CAD build for the part. Positions are in the model's coordinates, mm. Face numbers are marked on the shaded views. A direction names the side the tool comes from. Coordinates: 2 decimals unless noted, no trailing zeros. Order: outer loops, then holes, each group sorted by start corner. A loop starts at its lowest first (then second) coordinate and runs counter-clockwise, first axis right, second up. Notation, with made-up numbers: (-24, 86.5) - (30, 86.5) arc R17 ccw to (30, 108.5) - close; hole circle Ø1 at (-3.5, 30). An arc over 180 degrees is marked (long way). Write each question's results on one line, items separated by ' | '. Start each with the question number.
Q1. Which spindle directions (+Z, -Z, +X, -X, +Y, -Y) get a long thin tool onto all of the face, cutting with end or side? Do the marked faces 4, 5, 6, 7 and 8. Say none if no direction does.
Q2. Wall check: probe 1 along Y at (x, z) = (-32, 22.5); probe 2 along Z at (x, y) = (47, -12.5); probe 3 along X at (y, z) = (9, 4). Give the ranges that are in metal, low to high.
Q3. Pin check, flat tips, straight feed: P1, Ø20.5, axis at x = 36.5, y = -8.5, coming from the +Z side; P2, Ø5.5, axis at x = 15, z = 40, coming from the -Y side; P3, Ø5, axis at x = 22.5, z = 38, coming from the +Y side. Stop position of each tip, or through.
Q4. Band-saw the part on B-B, the plane y = -38. Write the cut outline in (x, z), then the cut area to 3 significant figures.
Q5. Band-saw the part on C-C, the plane z = 7. Count the separate pieces of the cut face and the enclosed holes in it, then the cut area to 3 significant figures.
Q6. Band-saw the part on A-A, the plane x = 12. Write the cut outline in (y, z) (3 decimals), then the cut area to 3 significant figures.
Q7. Pull direction X, two halves, no side cores. Call the marked faces 1, 2 and 3: released by +X, released by -X, zero draft, split by the parting line, or undercut.
Q8. Band-saw the part on D-D, the plane z = 82. Write the cut outline in (x, y).
```python
from build123d import *

# Parameters (mm, degrees)
F0_W         = 101.6
F0_H         = 76.2
F1_DEPTH     = 25.4
F2_R         = 15.875
F3_R         = 15.875
F4_R         = 15.875
F5_R         = 15.875
F7_D         = 15.875
F8_SIZE      = 6.35
F9_W         = 19.05
F9_H         = 63.5
F10_DEPTH    = 69.85
F12_DEPTH    = 25.4
F13_T1_DEPTH = 156.5315328508
F14_T1_DEPTH = 156.5315328508


# Not quite as in the source:
# - a fillet or chamfer that OpenCascade refuses, or shapes differently, is made with other operations: its cross-section is extruded or revolved along the edge and cut away or added


with BuildPart() as f1:
    # F0 (on Top) → F1 (new body)
    with BuildSketch(Plane.XY):
        with Locations((6.2353381336, -17.6054243982)):
            Rectangle(F0_W, F0_H)
    extrude(amount=F1_DEPTH)

    # F2
    f2_edges = [f1.edges().sort_by_distance(p)[0] for p in [
        (57.035338, -55.705424, 12.7),
    ]]
    fillet(f2_edges, radius=F2_R)

    # F3
    f3_edges = [f1.edges().sort_by_distance(p)[0] for p in [
        (-44.564662, -55.705424, 12.7),
    ]]
    fillet(f3_edges, radius=F3_R)

    # F4
    f4_edges = [f1.edges().sort_by_distance(p)[0] for p in [
        (-44.564662, 20.494576, 12.7),
    ]]
    fillet(f4_edges, radius=F4_R)

    # F5
    f5_edges = [f1.edges().sort_by_distance(p)[0] for p in [
        (57.035338, 20.494576, 12.7),
    ]]
    fillet(f5_edges, radius=F5_R)

    # F7 (through all)
    with Locations(Plane(origin=(0, 0, 0), x_dir=(1, 0, 0), z_dir=(0, 0, -1))):
        with Locations((-28.6896618664, 39.8304243982), (41.1603381336, 39.8304243982), (41.1603381336, -4.6195756018), (-28.6896618664, -4.6195756018)):
            Hole(F7_D / 2)

    # F8
    f8_edges = [f1.edges().sort_by_distance(p)[0] for p in [
        (6.235338, -55.705424, 25.4),
        (6.235338, 20.494576, 25.4),
        (52.385658, 15.844896, 25.4),
        (-39.914982, 15.844896, 25.4),
        (57.035338, -17.605424, 25.4),
        (-44.564662, -17.605424, 25.4),
        (52.385658, -51.055745, 25.4),
        (-39.914982, -51.055745, 25.4),
    ]]
    chamfer(f8_edges, length=F8_SIZE)

    # F9 (on face) → F10 (join)
    with BuildSketch(Plane.XY.offset(25.4)):
        with Locations((15.7603381336, -17.6054243982)):
            Rectangle(F9_W, F9_H)
    extrude(amount=F10_DEPTH)

    # F11 (on face) → F12 (cut)
    with BuildSketch(Plane(origin=(6.2353381336, 0, 0), x_dir=(0, -1, 0), z_dir=(-1, 0, 0))):
        with BuildLine():
            ThreePointArc((1.7304243982, 60.325), (17.6054243982, 44.45), (33.4804243982, 60.325))
            ThreePointArc((33.4804243982, 60.325), (17.6054243982, 76.2), (1.7304243982, 60.325))
        make_face()
        with BuildLine():
            ThreePointArc((1.7304243982, 60.325), (17.6054243982, 76.2), (33.4804243982, 60.325))
            Line((33.4804243982, 60.325), (33.4804243982, 95.25))
            Line((33.4804243982, 95.25), (1.7304243982, 95.25))
            Line((1.7304243982, 95.25), (1.7304243982, 60.325))
        make_face()
    extrude(amount=-F12_DEPTH, mode=Mode.SUBTRACT)

    # F13: fillet of radius 31.75 on 1 edges, made by hand

    # F13_s2 → F13_t1 (cut)
    with BuildSketch(Plane.YZ.offset(-62.5054282918)):
        with BuildLine():
            ThreePointArc((-33.4804243982, 95.25), (-45.1017309683, 83.6286934298), (-49.3554243982, 67.7536934298))
            Line((-49.3554243982, 67.7536934298), (-49.3554243982, 95.25))
            Line((-49.3554243982, 95.25), (-33.4804243982, 95.25))
        make_face()
    extrude(amount=F13_T1_DEPTH, mode=Mode.SUBTRACT)

    # F14: fillet of radius 31.75 on 1 edges, made by hand

    # F14_s2 → F14_t1 (cut)
    with BuildSketch(Plane.YZ.offset(-62.5054282918)):
        with BuildLine():
            ThreePointArc((14.1445756018, 67.7536934298), (9.890882172, 83.6286934298), (-1.7304243982, 95.25))
            Line((-1.7304243982, 95.25), (14.1445756018, 95.25))
            Line((14.1445756018, 95.25), (14.1445756018, 67.7536934298))
        make_face()
    extrude(amount=F14_T1_DEPTH, mode=Mode.SUBTRACT)


solid = f1.part
```
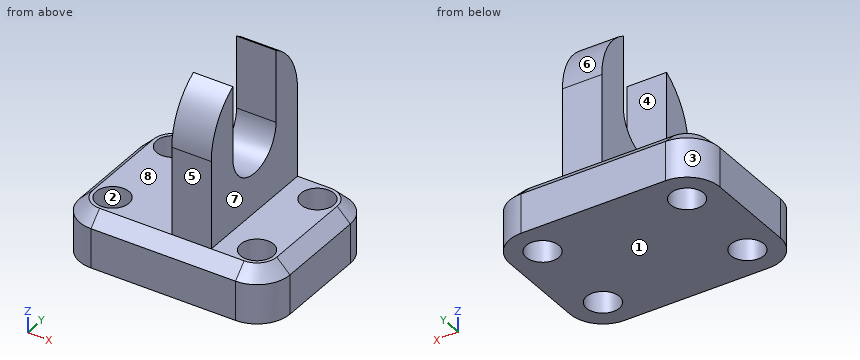
Results below:
1) face 4: +Z, +X, -X | face 5: +Z, +X, -X, -Y | face 6: +Z, +X, -X, +Y | face 7: +Z, +X, +Y, -Y | face 8: +Z, -X, +Y, -Y
2) probe 1: y = -51.81 to -47.04, -32.62 to -2.59, 11.83 to 16.6 | probe 2: z = 0 to 25.4 | probe 3: x = -43.95 to -35.31, -22.07 to 34.54, 47.78 to 56.42
3) P1: stops at z = 25.4 | P2: stops at y = -49.36 | P3: stops at y = 14.14
4) outline: (-44.56, 0) - (-36.41, 0) - (-36.41, 25.4) - (-38.21, 25.4) - (-44.56, 19.05) - close; (-20.97, 0) - (33.44, 0) - (33.44, 25.4) - (25.29, 25.4) - (25.29, 92.09) - (6.24, 92.09) - (6.24, 25.4) - (-20.97, 25.4) - close; (48.88, 0) - (57.04, 0) - (57.04, 19.05) - (50.69, 25.4) - (48.88, 25.4) - close | area: 3,030 mm²
5) separate pieces: 1 | enclosed holes: 4 | area: 6,730 mm²
6) outline: (-55.705, 0) - (20.495, 0) - (20.495, 19.05) - (14.145, 25.4) - (14.145, 67.754) arc R31.75 ccw to (-1.73, 95.25) - (-1.73, 60.325) arc R15.875 cw to (-33.48, 60.325) - (-33.48, 95.25) arc R31.75 ccw to (-49.355, 67.754) - (-49.355, 25.4) - (-55.705, 19.05) - close | area: 4,570 mm²
7) face 1: zero draft | face 2: undercut | face 3: released by -X
8) outline: (6.24, -45.98) - (25.29, -45.98) - (25.29, -33.48) - (6.24, -33.48) - close; (6.24, -1.73) - (25.29, -1.73) - (25.29, 10.77) - (6.24, 10.77) - close
